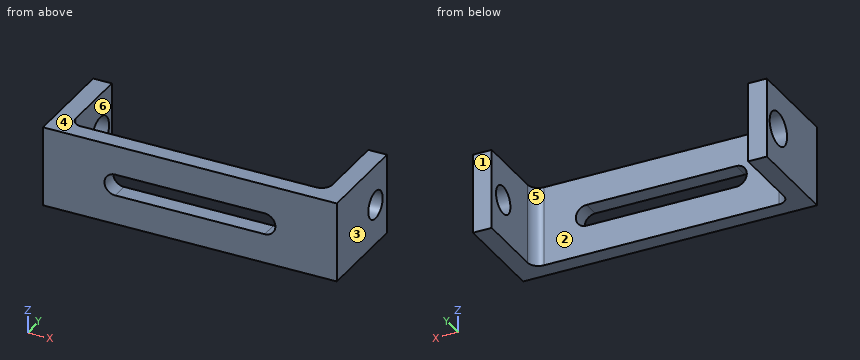
from build123d import *

# Parameters (mm, degrees)
SKETCH1_W           = 55
SKETCH1_H           = 15
BOSS_EXTRUDE1_DEPTH = 3.175
SKETCH2_W           = 3.5
SKETCH2_H           = 15
BOSS_EXTRUDE2_DEPTH = 15
FILLET1_R           = 2
CUT_EXTRUDE1_DEPTH  = 33.210246817
SKETCH4_R           = 2.6
CUT_EXTRUDE2_DEPTH  = 10
SKETCH5_R           = 3.15
CUT_EXTRUDE3_DEPTH  = 5


with BuildPart() as part:
    # Sketch1 → Boss-Extrude1 (new body)
    with BuildSketch(Plane(origin=(0, 0, 0), x_dir=(1, 0, 0), z_dir=(0, 1, 0))):
        Rectangle(SKETCH1_W, SKETCH1_H)
    extrude(amount=BOSS_EXTRUDE1_DEPTH)

    # Sketch2 → Boss-Extrude2 (add)
    with BuildSketch(Plane(origin=(0, 3.175, 0), x_dir=(1, 0, 0), z_dir=(0, 1, 0))):
        with Locations((-25.75, 0)):
            Rectangle(SKETCH2_W, SKETCH2_H)
        with Locations((25.75, 0)):
            Rectangle(SKETCH2_W, SKETCH2_H)
    extrude(amount=BOSS_EXTRUDE2_DEPTH)

    # Fillet1
    fillet1_edges = [part.edges().sort_by_distance(p)[0] for p in [
        (-24, 3.175, 0),
        (24, 3.175, 0),
    ]]
    fillet(fillet1_edges, radius=FILLET1_R)

    # Sketch3 → Cut-Extrude1 (cut, through all)
    with BuildSketch(Plane(origin=(0, 3.175, 0), x_dir=(1, 0, 0), z_dir=(0, 1, 0))):
        with BuildLine():
            Line((-14, 2), (14, 2))
            ThreePointArc((14, 2), (16, 0), (14, -2))
            Line((14, -2), (-14, -2))
            ThreePointArc((-14, -2), (-16, 0), (-14, 2))
        make_face()
    extrude(amount=-CUT_EXTRUDE1_DEPTH, mode=Mode.SUBTRACT)

    # Sketch4 → Cut-Extrude2 (cut)
    with BuildSketch(Plane(origin=(27.5, 0, 0), x_dir=(0, 0, -1), z_dir=(1, 0, 0))):
        with Locations((0, 14)):
            Circle(SKETCH4_R)
    extrude(amount=-CUT_EXTRUDE2_DEPTH, mode=Mode.SUBTRACT)

    # Sketch5 → Cut-Extrude3 (cut)
    with BuildSketch(Plane.ZY.offset(27.5)):
        with Locations((0, 14)):
            Circle(SKETCH5_R)
    extrude(amount=-CUT_EXTRUDE3_DEPTH, mode=Mode.SUBTRACT)


solid = part.part
For this review, take the finished solid that the model builds, in its own axes (mm). Face numbers are marked on the shaded views. A direction names the side the tool comes from. Round coordinates to 2 decimals unless told otherwise and drop trailing zeros. Order: outer loops, then holes, each group sorted by start corner. A loop starts at its lowest first (then second) coordinate and runs counter-clockwise, first axis right, second up. Notation, with made-up numbers: (-32.75, -4) -> (-27.75, -4) arc R19 ccw to (-27.75, 1) -> close; hole circle Ø9 at (11, 79.25). An arc over 180 degrees is marked (long way). Write item = value, one per line. Start each with the question number.
1) Tool access review of the marked faces 1 and 2: name each direction out of +Z, -Z, +X, -X, +Y, -Y from which nothing blocks a thin tool from reaching the whole face with its end or side.
2) Take a section at C-C on z = 0. State the section outline as (x, y) points (3 decimals).
3) Take a section at B-B on y = 8.75. State the section outline as (x, z) points, plus the area to 3 significant figures.
4) Insertion check: pin 1 (6 mm diameter, centred on y = 12, z = -0.5, fed in from -X); pin 2 (4.5 mm diameter, centred on y = 14, z = 0, fed in from +X). Each pin has a flat end and moves straight along its axis. Give the tip position at first contact, or say it passes through.
5) Take a section at A-A on x = 6.5. State the section outline as (y, z) points (3 decimals), plus the area to 3 significant figures.
6) To check wall thickness, follow line 1 (Y direction, x = -24.9, z = 0) (3 decimals); line 2 (X direction, y = 11.5, z = -3.25); line 3 (Y direction, x = 16, z = 4.25) (3 decimals). State the ranges of each line that lie inside material, in increasing order. Write a range as from..to.
7) The part is to be moulded in two halves that separate along X. For the marked faces 3, 4, 5 and 6, say which applies: +X half, -X half, draft (parallel to the pull), parting line (faces both ways), or undercut.
8) Take a section at D-D on y = 13.25. State the section outline as (x, z) points, plus the area to 3 significant figures.
Verdict:
q1.face_1 = +Z, -Z, +X, -X, +Y
q1.face_2 = +Z, -Z, +Y
q2.outline = (-27.5, 0) -> (-16, 0) -> (-16, 3.175) -> (-22, 3.175) arc R2 cw to (-24, 5.175) -> (-24, 10.85) -> (-27.5, 10.85) -> close; (-27.5, 17.15) -> (-24, 17.15) -> (-24, 18.175) -> (-27.5, 18.175) -> close; (16, 0) -> (27.5, 0) -> (27.5, 11.4) -> (24, 11.4) -> (24, 5.175) arc R2 cw to (22, 3.175) -> (16, 3.175) -> close; (24, 16.6) -> (27.5, 16.6) -> (27.5, 18.175) -> (24, 18.175) -> close
q3.outline = (-27.5, -7.5) -> (-24, -7.5) -> (-24, 7.5) -> (-27.5, 7.5) -> close; (24, -7.5) -> (27.5, -7.5) -> (27.5, 7.5) -> (24, 7.5) -> close
q3.area = 105 mm2
q4.pin_1 = -27.5
q4.pin_2 = through
q5.outline = (0, -7.5) -> (3.175, -7.5) -> (3.175, -2) -> (0, -2) -> close; (0, 2) -> (3.175, 2) -> (3.175, 7.5) -> (0, 7.5) -> close
q5.area = 34.9 mm2
q6.line_1 = 0..10.85, 17.15..18.175
q6.line_2 = -27.5..-24, 24..27.5
q6.line_3 = 0..3.175
q7.face_3 = +X half
q7.face_4 = draft
q7.face_5 = undercut
q7.face_6 = undercut
q8.outline = (-27.5, -7.5) -> (-24, -7.5) -> (-24, -3.06) -> (-27.5, -3.06) -> close; (-27.5, 3.06) -> (-24, 3.06) -> (-24, 7.5) -> (-27.5, 7.5) -> close; (24, -7.5) -> (27.5, -7.5) -> (27.5, -2.49) -> (24, -2.49) -> close; (24, 2.49) -> (27.5, 2.49) -> (27.5, 7.5) -> (24, 7.5) -> close
q8.area = 66.2 mm2
